```python
from build123d import *

# Parameters (mm, degrees)
PAD_DEPTH            = 1
PAD001_DEPTH         = 0.25
BODY_PLACEMENT_ANGLE = 45


with BuildPart() as part:
    # Sketch → Pad (new body)
    with BuildSketch(Plane.XY):
        with BuildLine():
            ThreePointArc((1.3228756555, -1.5), (0, 2), (-1.3228756555, -1.5))
            Line((-1.3228756555, -1.5), (1.3228756555, -1.5))
        make_face()
    extrude(amount=PAD_DEPTH)

    # Sketch001 → Revolution (revolve)
    with BuildSketch(Plane.YZ):
        with BuildLine():
            Line((0, 5.2), (0, 1))
            Line((0, 1), (-1.5, 1))
            Line((-1.5, 1), (-1.4264055883, 3.8104571954))
            ThreePointArc((0, 5.2), (-0.9956734038, 4.7951927894), (-1.4264055883, 3.8104571954))
        make_face()
    revolve(axis=Axis((0, 0, 0), (0, 0, 1)))

    # Sketch002 → Pad001 (join, symmetric)
    with BuildSketch(Plane.YZ):
        with BuildLine():
            Line((-0.325, 0), (-1.52, 0))
            Line((-1.52, 0), (-1.52, -0.4))
            ThreePointArc((-1.5869872981, -0.65), (-1.5370370869, -0.5294095226), (-1.52, -0.4))
            Line((-1.5869872981, -0.65), (-1.912076628, -1.2130712364))
            ThreePointArc((-1.912076628, -1.2130712364), (-2.0119770505, -1.4542521913), (-2.0460512242, -1.7130712364))
            Line((-2.0460512242, -1.7130712364), (-2.0460512242, -3.175))
            Line((-2.0460512242, -3.175), (-1.5460512242, -3.175))
            Line((-1.5460512242, -3.175), (-1.5460512242, -1.7130712364))
            ThreePointArc((-1.4790639261, -1.4630712364), (-1.5290141374, -1.5836617138), (-1.5460512242, -1.7130712364))
            Line((-1.1539745962, -0.9), (-1.4790639261, -1.4630712364))
            ThreePointArc((-1.1539745962, -0.9), (-1.0540741737, -0.6588190451), (-1.02, -0.4))
            Line((-0.325, -0.4), (-1.02, -0.4))
            Line((-0.325, 0), (-0.325, -0.4))
        make_face()
        with BuildLine():
            Line((0.325, 0), (1.52, 0))
            Line((1.52, 0), (1.52, -0.4))
            ThreePointArc((1.52, -0.4), (1.5370370869, -0.5294095226), (1.5869872981, -0.65))
            Line((1.5869872981, -0.65), (1.912076628, -1.2130712364))
            ThreePointArc((2.0460512242, -1.7130712364), (2.0119770505, -1.4542521913), (1.912076628, -1.2130712364))
            Line((2.0460512242, -1.7130712364), (2.0460512242, -3.175))
            Line((2.0460512242, -3.175), (1.5460512242, -3.175))
            Line((1.5460512242, -3.175), (1.5460512242, -1.7130712364))
            ThreePointArc((1.5460512242, -1.7130712364), (1.5290141374, -1.5836617138), (1.4790639261, -1.4630712364))
            Line((1.1539745962, -0.9), (1.4790639261, -1.4630712364))
            ThreePointArc((1.02, -0.4), (1.0540741737, -0.6588190451), (1.1539745962, -0.9))
            Line((0.325, -0.4), (1.02, -0.4))
            Line((0.325, 0), (0.325, -0.4))
        make_face()
    extrude(amount=PAD001_DEPTH, both=True)


with BuildPart() as part_1:
    # Body placement: moved
    add(part.part.moved(Location((-3.81, 0, 3.575))).rotate(Axis((-3.81, 0, 3.575), (0, 0, 1)), BODY_PLACEMENT_ANGLE))


with BuildPart() as part_2:
    # Clone008 placement: moved
    add(part_1.part.moved(Location((7.62, 0, 0.0445))))


solid = part_2.part
```
Check sheet for the modelled part. Datum: model origin and axes. Units: mm. A direction names the side the tool comes from. Round coordinates to 2 decimals unless told otherwise and drop trailing zeros. Loops run counter-clockwise (first coordinate to the right, second up) from the corner with the lowest first, then second, coordinate; pieces in that order, holes last. Notation, with made-up numbers: M 18,-36.5 L 75,-36.5 A29 cw 75,-10.5 Z; hole C 88,84 d6. An arc over 180 degrees is marked long. Answer as a JSON object with one key per item and string values.
1. Gauge pin test, flat end, axial feed: P1, Ø0.9, axis at x = 4.5, y = -0.5, coming from the -Z side. Record the tip position at first contact, or that the pin passes through.
Reply:
{"P1": "stops at z = 2.48"}
2. Section check A-A (z = 1.5). Record the boundary of the cut face in (x, y), plus the area to 3 significant figures.
Reply:
{"outline": "M 2.19,1.27 L 2.54,0.92 L 2.89,1.27 L 2.54,1.62 Z; M 4.73,-1.27 L 5.08,-1.62 L 5.43,-1.27 L 5.08,-0.92 Z", "area": "0.500 mm²"}
3. Section check C-C (z = 7.25). Record the boundary of the cut face in (x, y).
Reply:
{"outline": "C 3.81,0 d2.86"}
4. Access from +Z, -Z, +X, -X, +Y, -Y to the whole of each face (thin tool, end or side, straight path). Record for faces 1 (the flat face through (4.3, -0.5, 3.22)), 2 (the flat face through (5.143, -0.98, 2.392)), 3 (the flat face through (3.3, 0.5, 3.22)), 4 (the flat face through (4.79, -1.333, 2.392)), 5 (the conical face through (2.36, 0.19, 6.04)).
Reply:
{"face 1": "-Z, -X, +Y", "face 2": "-Z, +X, +Y", "face 3": "-Z, +X, -Y", "face 4": "-Z, -X, -Y", "face 5": "+Z"}
5. Section check B-B (z = 5.5). Record the boundary of the cut face in (x, y), plus the area to 3 significant figures.
Reply:
{"outline": "C 3.81,0 d2.95", "area": "6.85 mm²"}
6. Scan lines: line 1 (Z direction, x = 5.25, y = -0.6); line 2 (Y direction, x = 3.75, z = 8.5); line 3 (Z direction, x = 4.5, y = 0.8). Record each from-to range of solid material in increasing order.
Reply:
{"line 1": "z = 3.62 to 4.62", "line 2": "y = -0.9 to 0.9", "line 3": "z = 3.62 to 8.35"}
